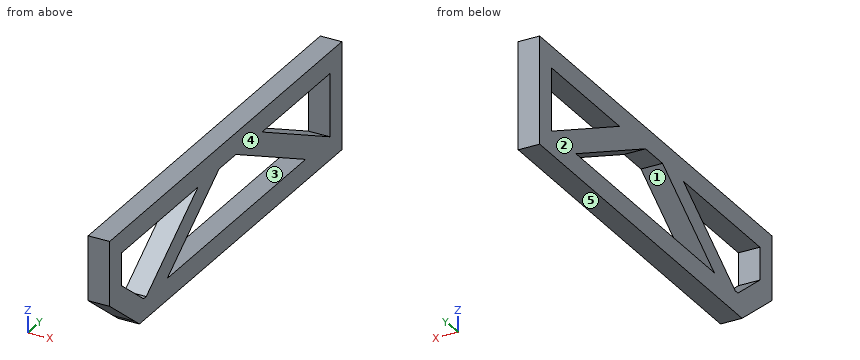
from build123d import *

# Parameters (mm, degrees)
F1_DEPTH = 20


with BuildPart() as f1:
    # F0 (on Right) → F1 (new body, symmetric)
    with BuildSketch(Plane.YZ):
        with BuildLine():
            Line((-304.9687541528, -20), (-368.9999965272, -20))
            Line((-368.9999965272, -20), (-284.617372716, -87.5060990489))
            ThreePointArc((-284.617372716, -87.5060990489), (-282.6313428058, -85.3648915743), (-280.3546556432, -83.5357442817))
            Line((-280.3546556432, -83.5357442817), (-246.2278264348, -60))
            Line((-246.2278264348, -60), (-254.9687541528, -60))
            Line((-254.9687541528, -60), (-304.9687541528, -20))
        make_face()
        Polygon((-175.7721666195, -60), (-233.7721666195, -100), (367.1707894712, -100), (289.1707894712, -60), align=None)
        Polygon((411.0000034728, 100), (64.8292174745, 100), (142.8292174745, 60), (371.0000034728, 60), (371.0000034728, -57.0106594863), (411.0000034728, -77.5234799992), align=None)
        with BuildLine():
            Line((64.8292174745, 100), (41.0000034728, 100))
            ThreePointArc((41.0000034728, 100), (40.4412866754, 95.3056941474), (38.7963527291, 90.8736670481))
            Line((38.7963527291, 90.8736670481), (99.0000034728, 60))
            Line((99.0000034728, 60), (142.8292174745, 60))
            Line((142.8292174745, 60), (64.8292174745, 100))
        make_face()
        with BuildLine():
            Line((99.0000034728, 60), (38.7963527291, 90.8736670481))
            ThreePointArc((38.7963527291, 90.8736670481), (36.0301930895, 86.8055541955), (32.3546625889, 83.5357442817))
            Line((32.3546625889, 83.5357442817), (22.5123293603, 76.747928262))
            Line((22.5123293603, 76.747928262), (55.1707894712, 60))
            Line((55.1707894712, 60), (99.0000034728, 60))
        make_face()
        Polygon((22.5123293603, 76.747928262), (-1.7721666195, 60), (55.1707894712, 60), align=None)
        with BuildLine():
            ThreePointArc((11.8736705209, 82.2036507437), (7.8055576683, 84.9698103834), (4.5357477545, 88.6453408839))
            Line((4.5357477545, 88.6453408839), (-36.9999965272, 60))
            Line((-36.9999965272, 60), (-1.7721666195, 60))
            Line((-1.7721666195, 60), (22.5123293603, 76.747928262))
            Line((22.5123293603, 76.747928262), (11.8736705209, 82.2036507437))
        make_face()
        with BuildLine():
            Line((1.0000034728, 100), (-14.2278264348, 100))
            Line((-14.2278264348, 100), (-72.2278264348, 60))
            Line((-72.2278264348, 60), (-36.9999965272, 60))
            Line((-36.9999965272, 60), (4.5357477545, 88.6453408839))
            ThreePointArc((4.5357477545, 88.6453408839), (1.9043872957, 94.0537875234), (1.0000034728, 100))
        make_face()
        with BuildLine():
            Line((21.0000034728, 100), (1.0000034728, 100))
            ThreePointArc((1.0000034728, 100), (1.9043872957, 94.0537875234), (4.5357477545, 88.6453408839))
            Line((4.5357477545, 88.6453408839), (21.0000034728, 100))
        make_face()
        with BuildLine():
            Line((38.7963527291, 90.8736670481), (21.0000034728, 100))
            Line((21.0000034728, 100), (4.5357477545, 88.6453408839))
            ThreePointArc((4.5357477545, 88.6453408839), (7.8055576683, 84.9698103834), (11.8736705209, 82.2036507437))
            Line((11.8736705209, 82.2036507437), (22.5123293603, 76.747928262))
            Line((22.5123293603, 76.747928262), (32.3546625889, 83.5357442817))
            ThreePointArc((32.3546625889, 83.5357442817), (36.0301930895, 86.8055541955), (38.7963527291, 90.8736670481))
        make_face()
        with BuildLine():
            Line((41.0000034728, 100), (21.0000034728, 100))
            Line((21.0000034728, 100), (38.7963527291, 90.8736670481))
            ThreePointArc((38.7963527291, 90.8736670481), (40.4412866754, 95.3056941474), (41.0000034728, 100))
        make_face()
        Polygon((-368.9999965272, 100), (-368.9999965272, 0), (-368.9999965272, -20), (-304.9687541528, -20), (-328.9999965272, -0.7750061005), (-328.9999965272, 60), (-72.2278264348, 60), (-14.2278264348, 100), align=None)
        Polygon((-210.9999965272, -60), (-268.9999965272, -100), (-233.7721666195, -100), (-175.7721666195, -60), align=None)
        with BuildLine():
            ThreePointArc((-280.3546556432, -83.5357442817), (-282.6313428058, -85.3648915743), (-284.617372716, -87.5060990489))
            Line((-284.617372716, -87.5060990489), (-268.9999965272, -100))
            Line((-268.9999965272, -100), (-210.9999965272, -60))
            Line((-210.9999965272, -60), (-246.2278264348, -60))
            Line((-246.2278264348, -60), (-280.3546556432, -83.5357442817))
        make_face()
        Polygon((-36.9999965272, 60), (-72.2278264348, 60), (-246.2278264348, -60), (-210.9999965272, -60), align=None)
        Polygon((-36.9999965272, 60), (-210.9999965272, -60), (-175.7721666195, -60), (-1.7721666195, 60), align=None)
        Polygon((55.1707894712, 60), (289.1707894712, -60), (333.0000034728, -60), (99.0000034728, 60), align=None)
        Polygon((142.8292174745, 60), (99.0000034728, 60), (333.0000034728, -60), (371.0000034728, -60), (371.0000034728, -57.0106594863), align=None)
        Polygon((289.1707894712, -60), (367.1707894712, -100), (411.0000034728, -100), (333.0000034728, -60), align=None)
        Polygon((333.0000034728, -60), (411.0000034728, -100), (411.0000034728, -77.5234799992), (371.0000034728, -57.0106594863), (371.0000034728, -60), align=None)
    extrude(amount=F1_DEPTH, both=True)


solid = f1.part
CAD build for the part. Positions are in the model's coordinates, mm. Face numbers are marked on the shaded views. A direction names the side the tool comes from. Round coordinates to 2 decimals unless told otherwise and drop trailing zeros. Loops run counter-clockwise (first coordinate to the right, second up) from the corner with the lowest first, then second, coordinate; pieces in that order, holes last. Notation, with made-up numbers: M 48.5,17.25 L 100.5,17.25 A11 ccw 100.5,25.25 Z; hole C 11.25,21 d7. An arc over 180 degrees is marked long. One line per question, with ' | ' between items. Start each with the question number.
Item 1: Pin check, flat tips, straight feed: pin 1 Ø8 at (x, z) = (-15, -46.5) entering from -Y (3 decimals); pin 2 Ø4 at (x, z) = (-4, -47) entering from -Y; pin 3 Ø10 at (x, z) = (-3.5, -33) entering from -Y. Stop position of each tip, or through.
Item 2: Cut at A-A, the plane y = 18.5. Write the cut outline in (x, z), plus the area to 3 significant figures.
Item 3: Wall check: line 1 (Y direction, x = 10, z = -12); line 2 (Z direction, x = 12.5, y = 206); line 3 (Y direction, x = 5, z = 6). Give the ranges that are in metal, low to high.
Item 4: Cut at C-C, the plane z = 7. Write the cut outline in (x, y).
Item 5: Two-plate mould, pull along Z, no slides. Class the marked faces 3, 4 and 5: pulls with the +Z half, pulls with the -Z half, needs draft (parallel to the pull), parting line crosses it, or undercut.
Item 6: Cut at B-B, the plane x = -14. Write the cut outline in (y, z) (3 decimals).
Item 7: Which spindle directions (+Z, -Z, +X, -X, +Y, -Y) get a long thin tool onto all of the face, cutting with end or side? Do the marked faces 1 and 2. Say none if no direction does.
Item 8: Cut at D-D, the plane y = 216. Write the cut outline in (x, z).
Responses:
1) pin 1: stops at y = -340.875 | pin 2: stops at y = -337.75 | pin 3: stops at y = -359
2) outline: M -20,-100 L 20,-100 L 20,-60 L -20,-60 Z; M -20,60 L 20,60 L 20,100 L -20,100 Z | area: 3,200 mm²
3) line 1: y = -369 to -314.97, -176.63 to -106.17, 195.57 to 283.23, 371 to 411 | line 2: z = -100 to -60, -17.35 to 27.6, 60 to 100 | line 3: y = -369 to -329, -150.53 to -80.07, 160.47 to 248.13, 371 to 411
4) outline: M -20,-369 L 20,-369 L 20,-329 L -20,-329 Z; M -20,-149.08 L 20,-149.08 L 20,-78.62 L -20,-78.62 Z; M -20,158.52 L 20,158.52 L 20,246.18 L -20,246.18 Z; M -20,371 L 20,371 L 20,411 L -20,411 Z
5) face 3: undercut | face 4: needs draft | face 5: pulls with the -Z half
6) outline: M -369,-20 L -269,-100 L 411,-100 L 411,100 L -369,100 Z; hole M -329,-0.775 L -254.969,-60 L -246.228,-60 L -72.228,60 L -329,60 Z; hole M -175.772,-60 L 289.171,-60 L 55.171,60 L -1.772,60 Z; hole M 142.829,60 L 371,-57.011 L 371,60 Z
7) face 1: +X, -X | face 2: +Z, -Z, -X, +Y, -Y
8) outline: M -20,-100 L 20,-100 L 20,-60 L -20,-60 Z; M -20,-22.48 L 20,-22.48 L 20,22.48 L -20,22.48 Z; M -20,60 L 20,60 L 20,100 L -20,100 Z
